Can you work these out from the model? Positions are in its coordinate system, mm. Face numbers are marked on the shaded views. A direction names the side the tool comes from. Give positions to 0.01 mm unless a question says otherwise; leave off trailing zeros. Order: outer loops, then holes, each group sorted by start corner. A loop starts at its lowest first (then second) coordinate and runs counter-clockwise, first axis right, second up.
Item 1: I'm going to push flat-ended pins straight in: pin 1 Ø1 at (x, y) = (-6, 0.5) entering from -Z; pin 2 Ø3 at (x, z) = (2, 24.5) entering from +Y; pin 3 Ø1.5 at (y, z) = (-24.5, -14) entering from +X; pin 4 Ø12 at (x, z) = (11, -22.5) entering from +Y. Where does each tip first touch, or does it pass through?
Item 2: I want a section at A-A, the plane y = 0. Write out the boundary of the cut face in (x, z), then the cut area to 3 significant figures.
Item 3: I want a section at C-C, the plane x = 12. Write out the boundary of the cut face in (y, z), then the cut area to 3 significant figures.
Item 4: I want a section at D-D, the plane z = -35. Write out the boundary of the cut face in (x, y).
Item 5: Which directions (+Z, -Z, +X, -X, +Y, -Y) give clear straight access to the entire face, cutting with the end or side of a thin tool? Please do the marked faces 1, 2 and 3.
Item 6: If I drill on line 1 along X through (y, z) = (-20.5, 33); line 2 along X through (y, z) = (-17, -25); line 3 along Y through (x, z) = (-6.5, -25), over which ranges is the centre line in solid material (lowest first)?
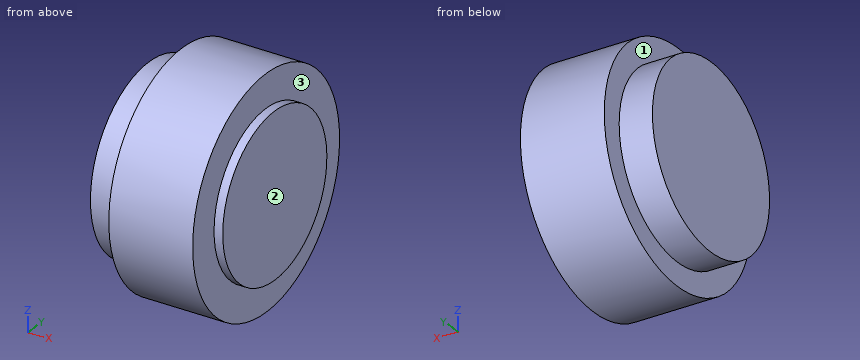
Autodesk Inventor part; units mm, degrees
ref_plane "YZ Plane" through (0, 0, 0) normal (1, 0, 0) x (0, 1, 0)
ref_plane "XZ Plane" through (0, 0, 0) normal (0, 1, 0) x (-1, 0, 0)
ref_plane "XY Plane" through (0, 0, 0) normal (0, 0, 1) x (1, 0, 0)
sketch "Sketch1" plane through (0, 0, 0) normal (1, 0, 0) x (0, 1, 0)
  circle A0 centre (0, 0) radius 31.5
  circle A1 centre (0, 0) radius 39.5
  dimension "d0" = 79
  dimension "d1" = 63
extrude "Extrusion1" add sketch "Sketch1" against normal blind 11.5 contours A0
extrude "Extrusion2" add sketch "Sketch1" along normal blind 29 contours A0 | A1
sketch "Sketch2" plane through (29, 0, 0) normal (1, 0, 0) x (0, 0, -1)
  circle A0 centre (0, 0) radius 28
  dimension "d12" = 56
extrude "Extrusion3" add sketch "Sketch2" along normal blind 3
properties part number "motor"
Results list:
1. pin 1: stops at z = -31.5
1. pin 2: stops at y = 32.11
1. pin 3: stops at x = 32
1. pin 4: stops at y = 35.89
2. outline: (-11.5, -31.5) - (0, -31.5) - (0, -39.5) - (29, -39.5) - (29, -28) - (32, -28) - (32, 28) - (29, 28) - (29, 39.5) - (0, 39.5) - (0, 31.5) - (-11.5, 31.5) - close
2. area: 3,180 mm2
3. outline: circle Ø79 at (0, 0)
3. area: 4,900 mm2
4. outline: (0, -18.31) - (29, -18.31) - (29, 18.31) - (0, 18.31) - close
5. face 1: -X
5. face 2: +Z, -Z, +X, +Y, -Y
5. face 3: +X
6. line 1: x = 0 to 29
6. line 2: x = -11.5 to 29
6. line 3: y = -19.16 to 19.16
